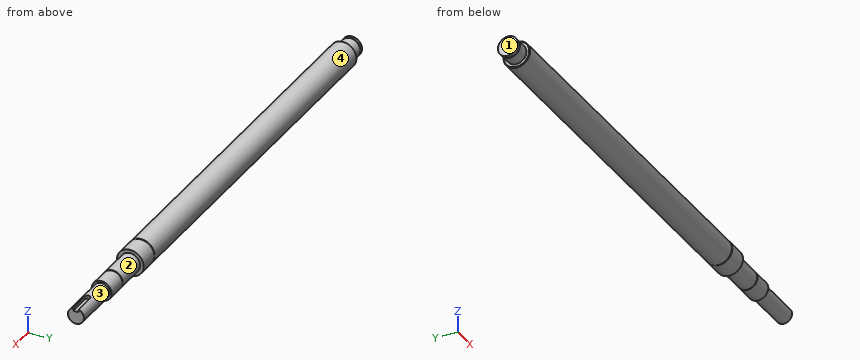
from build123d import *

# Parameters (mm, degrees)
F0_R      = 7.5
F1_DEPTH  = 9
F2_R      = 7.15
F3_DEPTH  = 1.15
F4_R      = 7.5
F5_DEPTH  = 1.85
F6_R      = 10
F7_DEPTH  = 283
F8_SIZE   = 0.5
F9_R      = 10
F10_DEPTH = 15
F11_R     = 7.5
F12_DEPTH = 25
F13_SIZE  = 0.5
F14_R     = 7.5
F15_DEPTH = 15
F16_R     = 6
F17_DEPTH = 36
F19_W     = 18
F19_H     = 4
F20_DEPTH = 2.5
F21_R     = 1.9999


# Not quite as in the source:
# - a fillet or chamfer is up to 0.001 mm smaller than in the source, because OpenCascade refuses the exact size


with BuildPart() as f1:
    # F0 (on Right) → F1 (new body)
    with BuildSketch(Plane.YZ):
        Circle(F0_R)
    extrude(amount=-F1_DEPTH)

    # F2 (on face) → F3 (join)
    with BuildSketch(Plane(origin=(-9, 0, 0), x_dir=(0, -1, 0), z_dir=(-1, 0, 0))):
        Circle(F2_R)
    extrude(amount=F3_DEPTH)

    # F4 (on face) → F5 (join)
    with BuildSketch(Plane(origin=(-10.15, 0, 0), x_dir=(0, -1, 0), z_dir=(-1, 0, 0))):
        Circle(F4_R)
    extrude(amount=F5_DEPTH)

    # F6 (on Right) → F7 (join)
    with BuildSketch(Plane.YZ):
        Circle(F6_R)
    extrude(amount=F7_DEPTH)

    # F8
    f8_edges = [f1.edges().sort_by_distance(p)[0] for p in [
        (283, -10, 0),
        (0, -10, 0),
    ]]
    chamfer(f8_edges, length=F8_SIZE)

    # F9 (on face) → F10 (join)
    with BuildSketch(Plane.YZ.offset(283)):
        Circle(F9_R)
    extrude(amount=F10_DEPTH)

    # F11 (on face) → F12 (join)
    with BuildSketch(Plane.YZ.offset(298)):
        Circle(F11_R)
    extrude(amount=F12_DEPTH)

    # F13
    f13_edges = [f1.edges().sort_by_distance(p)[0] for p in [
        (323, -7.5, 0),
    ]]
    chamfer(f13_edges, length=F13_SIZE)

    # F14 (on face) → F15 (join)
    with BuildSketch(Plane.YZ.offset(323)):
        Circle(F14_R)
    extrude(amount=F15_DEPTH)

    # F16 (on face) → F17 (join)
    with BuildSketch(Plane.YZ.offset(338)):
        Circle(F16_R)
    extrude(amount=F17_DEPTH)

    # F19 (on offset) → F20 (cut)
    with BuildSketch(Plane.XY.offset(6)):
        with Locations((365, 0)):
            Rectangle(F19_W, F19_H)
    extrude(amount=-F20_DEPTH, mode=Mode.SUBTRACT)

    # F21 (radius 2 in the source; OpenCascade refuses exactly that, so slightly less here)
    f21_edges = [f1.edges().sort_by_distance(p)[0] for p in [
        (356, 2, 4.578427),
        (356, -2, 4.578427),
    ]]
    fillet(f21_edges, radius=F21_R)


solid = f1.part
Source: CAD feature listing. Evaluate the final solid. Frame: model axes, mm. Face numbers are marked on the shaded views. A direction names the side the tool comes from. Round coordinates to 2 decimals unless told otherwise and drop trailing zeros. Order: outer loops, then holes, each group sorted by start corner. A loop starts at its lowest first (then second) coordinate and runs counter-clockwise, first axis right, second up. Notation, with made-up numbers: (27, -35.5) - (59, -35.5) arc R16 ccw to (59, -14.5) - close; hole circle Ø5 at (40.5, -18.75). An arc over 180 degrees is marked (long way). Use a Markdown table: item, result. Add a question column.
1. Section query A-A (x = 264). Return the cut outline in (y, z), then the cut area to 3 significant figures.
2. Set-up query: the marked faces 3 and 4. Return all of +Z, -Z, +X, -X, +Y, -Y with unobstructed straight access to the full face (end or side cutting, diameter ignored); none if empty.
3. Section query B-B (x = 343.5). Return the cut outline in (y, z).
4. First-contact query: pin 1 (3 mm diameter, centred on x = 328.5, y = -3.5, fed in from -Z); pin 2 (5 mm diameter, centred on x = 318, z = -6, fed in from -Y); pin 3 (1.1 mm diameter, centred on x = 364.5, z = 4.5, fed in from +Y). Flat tips, straight axial feed; report the tip coordinate or a pass-through.
5. Mould query, pull axis Z, two halves, no side actions, for the marked faces 1 and 2. Classes: +Z half, -Z half, draft (parallel to the pull), parting line (faces both ways), or undercut.
6. Line query: probe 1 along X at (y, z) = (-2.5, -7); probe 2 along X at (y, z) = (7.5, 3); probe 3 along Z at (x, y) = (245.5, -0.5). Output: solid intervals per line, ascending.
Derived:
| question | item | result |
|---|---|---|
| 1 | outline | circle Ø20 at (0, 0) |
| 1 | area | 314 mm2 |
| 2 | face 3 | +X |
| 2 | face 4 | +X, -X |
| 3 | outline | circle Ø12 at (0, 0) |
| 4 | pin 1 | z = -7.23 |
| 4 | pin 2 | y = -6.63 |
| 4 | pin 3 | y = 4.52 |
| 5 | face 1 | draft |
| 5 | face 2 | parting line |
| 6 | probe 1 | -12 to -10.15, -9 to 322.57, 323 to 338 |
| 6 | probe 2 | 0 to 298 |
| 6 | probe 3 | -9.99 to 9.99 |
